```python
from build123d import *

# Parameters (mm, degrees)
SKETCH1_W                = 40
SKETCH1_H                = 48
BOSS_EXTRUDE1_DEPTH      = 4
BOSS_EXTRUDE2_DEPTH      = 11.15
BOSS_EXTRUDE2_DEPTH_BACK = 4
SKETCH5_W                = 40
SKETCH5_H                = 5.225
SKETCH5_W_2              = 18
SKETCH5_H_2              = 5
SKETCH5_H_3              = 6
FILLET1_R                = 4
SKETCH6_R                = 1.35
CUT_EXTRUDE4_DEPTH       = 58.214705278
CHAMFER2_SIZE            = 2
SKETCH7_W                = 40
SKETCH7_H                = 6.5
CUT_EXTRUDE5_DEPTH       = 3
FILLET2_R                = 3
CHAMFER3_SIZE            = 3
CHAMFER3_SIZE2           = 1
CHAMFER4_SIZE            = 3
CHAMFER4_SIZE2           = 0.5
CUT_EXTRUDE6_DEPTH       = 10
CUT_EXTRUDE6_DEPTH_BACK  = 10
CUT_EXTRUDE8_REACH       = 66.292
SKETCH12_R               = 3
SKETCH13_R               = 1.5
CUT_EXTRUDE10_DEPTH      = 10.275
CUT_EXTRUDE7_DEPTH       = 1.25
CUT_EXTRUDE7_DEPTH_BACK  = 1.25


with BuildPart() as part:
    # Sketch1 → Boss-Extrude1 (new body)
    with BuildSketch(Plane.XY):
        with Locations((20, 14)):
            Rectangle(SKETCH1_W, SKETCH1_H)
    extrude(amount=BOSS_EXTRUDE1_DEPTH)

    # Sketch5 → Boss-Extrude2 (add, two sides: drawn at the far end of the back side and taken through both)
    with BuildSketch(Plane.XY.offset(4).offset(-BOSS_EXTRUDE2_DEPTH_BACK)):
        Polygon((0.9, 8.125), (0, 8.125), (0, 15.5), (40, 15.5), (40, 8.225), (28, 8.225), (27.025, 10.5), (11.081237185, 10.5), (9.763380042, 7.425), (8.800403155, 7.425), (8.500403155, 8.125), (7.531690021, 8.125), (7.231690021, 7.425), (6.221941609, 7.425), (5.921941609, 8.125), (5, 8.125), (4.7, 7.425), (3.7, 7.425), (3.4, 8.125), (2.5, 8.125), (2.2, 7.425), (1.2, 7.425), align=None)
        with Locations((20, 3.6125)):
            Rectangle(SKETCH5_W, SKETCH5_H)
        with Locations((20, -7.5)):
            Rectangle(SKETCH5_W_2, SKETCH5_H_2)
        with Locations((20, 35)):
            Rectangle(SKETCH5_W, SKETCH5_H_3)
    extrude(amount=BOSS_EXTRUDE2_DEPTH + BOSS_EXTRUDE2_DEPTH_BACK)

    # Fillet1
    fillet1_edges = [part.edges().sort_by_distance(p)[0] for p in [
        (20, 1, 4),
        (20, 32, 4),
    ]]
    fillet(fillet1_edges, radius=FILLET1_R)

    # Sketch6 → Cut-Extrude4 (cut, through all)
    with BuildSketch(Plane.XY.offset(15.15)):
        with Locations((7.5, 35)):
            Circle(SKETCH6_R)
        with Locations((7.5, 12)):
            Circle(SKETCH6_R)
        with Locations((32.5, 35)):
            Circle(SKETCH6_R)
        with Locations((32.5, 12)):
            Circle(SKETCH6_R)
    extrude(amount=-CUT_EXTRUDE4_DEPTH, mode=Mode.SUBTRACT)

    # Chamfer2
    chamfer2_edges = [part.edges().sort_by_distance(p)[0] for p in [
        (40, 8.225, 9.575),
        (0, 15.5, 9.575),
        (40, 15.5, 9.575),
    ]]
    chamfer(chamfer2_edges, length=CHAMFER2_SIZE)

    # Sketch7 → Cut-Extrude5 (cut)
    with BuildSketch(Plane.XY.offset(4)):
        with Locations((20, 18.75)):
            Rectangle(SKETCH7_W, SKETCH7_H)
    extrude(amount=-CUT_EXTRUDE5_DEPTH, mode=Mode.SUBTRACT)

    # Fillet2
    fillet2_edges = [part.edges().sort_by_distance(p)[0] for p in [
        (20, 15.5, 1),
        (20, 22, 1),
    ]]
    fillet(fillet2_edges, radius=FILLET2_R - 0.0001)  # a hair under: the kernel refuses the full size

    # Chamfer3
    chamfer3_edges = [part.edges().sort_by_distance(p)[0] for p in [
        (4.2, 7.425, 15.15),
    ]]
    chamfer3_side = [part.faces().sort_by_distance(p)[0] for p in [
        (4.2, 7.425, 9.575),
    ]]
    chamfer(chamfer3_edges, length=CHAMFER3_SIZE, length2=CHAMFER3_SIZE2, reference=chamfer3_side[0])

    # Chamfer4
    chamfer4_edges = [part.edges().sort_by_distance(p)[0] for p in [
        (20, 6.225, 15.15),
    ]]
    chamfer4_side = [part.faces().sort_by_distance(p)[0] for p in [
        (20, 6.225, 9.575),
    ]]
    chamfer(chamfer4_edges, length=CHAMFER4_SIZE, length2=CHAMFER4_SIZE2, reference=chamfer4_side[0])

    # Sketch8 → Cut-Extrude6 (cut, two sides: drawn at the far end of the back side and taken through both)
    with BuildSketch(Plane(origin=(20, 0, 0), x_dir=(0, 0, -1), z_dir=(1, 0, 0)).offset(-CUT_EXTRUDE6_DEPTH_BACK)):
        with BuildLine():
            Line((-9, 34.15), (-18.856272107, 34.15))
            Line((-18.856272107, 34.15), (-18.856272107, 21.85))
            Line((-18.856272107, 21.85), (-9, 21.85))
            ThreePointArc((-9, 21.85), (-2.85, 28), (-9, 34.15))
        make_face()
        with BuildLine():
            Line((-18.856272107, -10.437196649), (-18.856272107, -3.158858698))
            Line((-18.856272107, -3.158858698), (-13.348706704, 2.348706704))
            ThreePointArc((-13.348706704, 2.348706704), (-3.318140875, 0.353503109), (-9, -8.15))
            Line((-9, -8.15), (-9, -10.437196649))
            Line((-9, -10.437196649), (-18.856272107, -10.437196649))
        make_face()
    extrude(amount=CUT_EXTRUDE6_DEPTH + CUT_EXTRUDE6_DEPTH_BACK, mode=Mode.SUBTRACT)

    # Cut-Extrude8: up to this face of the body (flat: up to its plane)
    cut_extrude8_end = Plane(part.part.faces().sort_by_distance((20, 15.5, 9.574944444))[0])
    # Sketch12 → Cut-Extrude8 (cut, up to the picked face)
    with BuildSketch(Plane(origin=(0, 38, 0), x_dir=(1, 0, 0), z_dir=(0, 1, 0)), mode=Mode.PRIVATE) as cut_extrude8_sk1:
        with Locations(Location((15.4, -9, 0), (0, 0, 270))):
            Circle(SKETCH12_R)
    cut_extrude8_tool1 = split(extrude(cut_extrude8_sk1.sketch, amount=-CUT_EXTRUDE8_REACH, mode=Mode.PRIVATE), bisect_by=cut_extrude8_end, keep=Keep.BOTH, mode=Mode.PRIVATE)
    add(cut_extrude8_tool1.solids().sort_by(Axis((15.4, 38, 9), (0, -1, 0)))[0], mode=Mode.SUBTRACT)

    # Sketch13 → Cut-Extrude10 (cut)
    with BuildSketch(Plane(origin=(0, 15.5, 0), x_dir=(1, 0, 0), z_dir=(0, 1, 0))):
        with Locations(Location((15.4, -9, 0), (0, 0, 180))):
            Circle(SKETCH13_R)
    extrude(amount=-CUT_EXTRUDE10_DEPTH, mode=Mode.SUBTRACT)

    # Sketch9 → Cut-Extrude7 (cut, two sides: drawn at the far end of the back side and taken through both)
    with BuildSketch(Plane.XZ.offset(-13).offset(-CUT_EXTRUDE7_DEPTH_BACK)):
        Polygon((12.5, 16.815347994), (18.3, 16.815347994), (18.3, 7.325684219), (15.4, 5.651368439), (12.5, 7.325684219), align=None)
    extrude(amount=CUT_EXTRUDE7_DEPTH + CUT_EXTRUDE7_DEPTH_BACK, mode=Mode.SUBTRACT)


solid = part.part
```
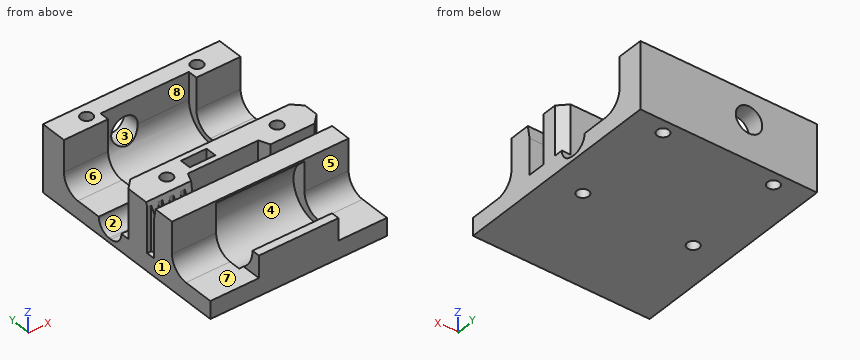
Build history of the part. All positions in model axes, mm. Face numbers are marked on the shaded views. A direction names the side the tool comes from. Round coordinates to 2 decimals unless told otherwise and drop trailing zeros. Order: outer loops, then holes, each group sorted by start corner. A loop starts at its lowest first (then second) coordinate and runs counter-clockwise, first axis right, second up. Notation, with made-up numbers: (38, -29) -> (57, -29) arc R10 cw to (57, -16) -> close; hole circle Ø10 at (7.5, -30.5). An arc over 180 degrees is marked (long way). Answer in a Markdown table with one row per item.
1) Pin check, flat tips, straight feed: P1, Ø1.1, axis at x = 2, z = 7, coming from the -Y side; P2, Ø9, axis at x = 18, z = 10.5, coming from the -Y side; P3, Ø0.8, axis at x = 9, z = 8, coming from the -Y side; P4, Ø1.3, axis at y = -7.5, z = 7, coming from the +X side. Stop position of each tip, or through.
Values:
| item | result |
|---|---|
| P1 | y = 0.69 |
| P2 | y = -10 |
| P3 | y = 0.98 |
| P4 | x = 29 |
2) Band-saw the part on A-A on y = 35. Give the cut face in (x, z).
Values:
| item | result |
|---|---|
| outline | (0, 0) -> (6.15, 0) -> (6.15, 15.15) -> (0, 15.15) -> close; (8.85, 0) -> (31.15, 0) -> (31.15, 15.15) -> (8.85, 15.15) -> close; (33.85, 0) -> (40, 0) -> (40, 15.15) -> (33.85, 15.15) -> close; hole circle Ø6 at (15.4, 9) |
3) Which spindle directions (+Z, -Z, +X, -X, +Y, -Y) get a long thin tool onto all of the face, cutting with end or side? Do the marked faces 5, 6, 7 and 8. Say none if no direction does.
Values:
| item | result |
|---|---|
| face 5 | +Z, +X, -X, -Y |
| face 6 | +Z, +X, -X |
| face 7 | +Z, -X, -Y |
| face 8 | +Z |
4) Wall check: L1, parallel to Y at x = 32.5, z = 8.75 (3 decimals); L2, parallel to Z at x = 15.4, y = 15.05; L3, parallel to Y at x = 34.5, z = 9 (3 decimals). Give the ranges that are in metal, low to high.
Values:
| item | result |
|---|---|
| L1 | 1 to 6.225, 8.225 to 10.65, 13.35 to 15.5, 32 to 33.65, 36.35 to 38 |
| L2 | 0 to 7.5, 10.5 to 15.15 |
| L3 | 1 to 6.225, 8.225 to 15.5, 32 to 38 |
5) Mould opens along X. For the marked faces 1, 2, 3 and 4 say: released by +X, released by -X, zero draft, split by the parting line, or undercut.
Values:
| item | result |
|---|---|
| face 1 | released by -X |
| face 2 | zero draft |
| face 3 | undercut |
| face 4 | undercut |
6) Band-saw the part on C-C on z = 2.25. Give the cut face in (x, y), and give its area (3 significant figures).
Values:
| item | result |
|---|---|
| outline | (0, -10) -> (40, -10) -> (40, 16.06) -> (0, 16.06) -> close; (0, 21.44) -> (40, 21.44) -> (40, 38) -> (0, 38) -> close; hole circle Ø2.7 at (7.5, 12); hole circle Ø2.7 at (7.5, 35); hole circle Ø2.7 at (32.5, 12); hole circle Ø2.7 at (32.5, 35) |
| area | 1,680 mm2 |
7) Band-saw the part on B-B on x = 32.5. Give the number of separate pieces and of enclosed holes in the cut face, and give its area (3 significant figures).
Values:
| item | result |
|---|---|
| separate pieces | 3 |
| enclosed holes | 0 |
| area | 307 mm2 |
